Can you work these out from the model? Positions are in its coordinate system, mm. A direction names the side the tool comes from. Round coordinates to 2 decimals unless told otherwise and drop trailing zeros. Loops run counter-clockwise (first coordinate to the right, second up) from the corner with the lowest first, then second, coordinate; pieces in that order, holes last.
(1) Thinking about a two-plate mould opening in X: for faces 1 (the face through (-13, 3, -69.85)), 2 (the face through (-95.25, 3, -63)), 3 (the face through (82.55, 3, 67)), which applies, released by +X, released by -X, zero draft, split by the parting line, or undercut?
(2) If I drill on line 1 along Z through (x, y) = (-29.5, 5.5); line 2 along X through (y, z) = (4.25, -48.5), over which ranges is the centre line in solid material (lowest first)?
(3) I want a section at A-A on x = 79. Write out the boundary of the cut face in (y, z).
(4) I want a section at B-B on z = 24. Write out the boundary of the cut face in (x, y).
(5) Which directions (+Z, -Z, +X, -X, +Y, -Y) give clear straight access to the entire face, cutting with the end or side of a thin tool? Please do faces 4 (the face through (-69.85, 3, 67)), 5 (the face through (6.35, 3, -67)), 6 (the face through (92, 3, -19.05)), 7 (the face through (-92, 3, 31.75)).
(6) Will this pin go through, and if not, where does the flat tip stop? pin 1 Ø3 at (x, y) = (-29, 5.5) entering from +Z.
from build123d import *

# Parameters (mm, degrees)
SKETCH1_W                   = 190.5
SKETCH1_H                   = 139.7
BOSS_EXTRUDE1_DEPTH         = 6.35
SKETCH2_W                   = 12.7
SKETCH2_H                   = 12.7
CUT_EXTRUDE1_DEPTH          = 6.35
LPATTERN1_COUNT             = 4
LPATTERN1_PITCH             = 25.4
LPATTERN2_COUNT             = 4
LPATTERN2_PITCH             = 25.4
CIRPATTERN1_COUNT           = 2
CIRPATTERN1_COPY_1_SKETCH_W = 12.7
CIRPATTERN1_COPY_1_SKETCH_H = 12.7
CIRPATTERN1_COPY_1_DEPTH    = 6.35
CIRPATTERN1_COPY_2_SKETCH_W = 12.7
CIRPATTERN1_COPY_2_SKETCH_H = 12.7
CIRPATTERN1_COPY_2_DEPTH    = 6.35
CIRPATTERN1_COPY_3_SKETCH_W = 12.7
CIRPATTERN1_COPY_3_SKETCH_H = 12.7
CIRPATTERN1_COPY_3_DEPTH    = 6.35
CIRPATTERN1_COPY_4_SKETCH_W = 12.7
CIRPATTERN1_COPY_4_SKETCH_H = 12.7
CIRPATTERN1_COPY_4_DEPTH    = 6.35
CIRPATTERN1_COPY_5_SKETCH_W = 12.7
CIRPATTERN1_COPY_5_SKETCH_H = 12.7
CIRPATTERN1_COPY_5_DEPTH    = 6.35
CIRPATTERN1_COPY_6_SKETCH_W = 12.7
CIRPATTERN1_COPY_6_SKETCH_H = 12.7
CIRPATTERN1_COPY_6_DEPTH    = 6.35
SKETCH3_W                   = 12.7
SKETCH3_H                   = 12.7
CUT_EXTRUDE2_DEPTH          = 6.35
LPATTERN3_COUNT             = 3
LPATTERN3_PITCH             = 25.4
LPATTERN4_COUNT             = 3
LPATTERN4_PITCH             = 25.4
CIRPATTERN2_COUNT           = 2
CIRPATTERN2_COPY_1_SKETCH_W = 12.7
CIRPATTERN2_COPY_1_SKETCH_H = 12.7
CIRPATTERN2_COPY_1_DEPTH    = 6.35
CIRPATTERN2_COPY_2_SKETCH_W = 12.7
CIRPATTERN2_COPY_2_SKETCH_H = 12.7
CIRPATTERN2_COPY_2_DEPTH    = 6.35
CIRPATTERN2_COPY_3_SKETCH_W = 12.7
CIRPATTERN2_COPY_3_SKETCH_H = 12.7
CIRPATTERN2_COPY_3_DEPTH    = 6.35
CIRPATTERN2_COPY_4_SKETCH_W = 12.7
CIRPATTERN2_COPY_4_SKETCH_H = 12.7
CIRPATTERN2_COPY_4_DEPTH    = 6.35


with BuildPart() as part:
    # Sketch1 → Boss-Extrude1 (new body)
    with BuildSketch(Plane(origin=(0, 0, 0), x_dir=(1, 0, 0), z_dir=(0, 1, 0))):
        Rectangle(SKETCH1_W, SKETCH1_H)
    extrude(amount=BOSS_EXTRUDE1_DEPTH)

    # Sketch2 → Cut-Extrude1 (cut)
    with BuildSketch(Plane(origin=(0, 6.35, 0), x_dir=(1, 0, 0), z_dir=(0, 1, 0))):
        with Locations((0, 69.85)):
            Rectangle(SKETCH2_W, SKETCH2_H)
    cut_extrude1 = extrude(amount=-CUT_EXTRUDE1_DEPTH, mode=Mode.SUBTRACT)

    # LPattern1: Cut-Extrude1 ×4
    with Locations(*[(-i * LPATTERN1_PITCH, 0, 0) for i in range(1, LPATTERN1_COUNT)]):
        add(cut_extrude1, mode=Mode.SUBTRACT)

    # LPattern2: Cut-Extrude1 ×4
    with Locations(*[(i * LPATTERN2_PITCH, 0, 0) for i in range(1, LPATTERN2_COUNT)]):
        add(cut_extrude1, mode=Mode.SUBTRACT)

    # CirPattern1: Cut-Extrude1 ×2 about axis
    cirpattern1_axis = Axis((0, 0, 0), (0, 1, 0))
    for i in range(1, CIRPATTERN1_COUNT):
        add(cut_extrude1.rotate(cirpattern1_axis, i * 360 / CIRPATTERN1_COUNT), mode=Mode.SUBTRACT)

    # CirPattern1 copy 1 sketch → CirPattern1 copy 1 (cut)
    with BuildSketch(Plane(origin=(25.4, 6.35, 0), x_dir=(-1, 0, 0), z_dir=(0, 1, 0))):
        with Locations((0, 69.85)):
            Rectangle(CIRPATTERN1_COPY_1_SKETCH_W, CIRPATTERN1_COPY_1_SKETCH_H)
    extrude(amount=-CIRPATTERN1_COPY_1_DEPTH, mode=Mode.SUBTRACT)

    # CirPattern1 copy 2 sketch → CirPattern1 copy 2 (cut)
    with BuildSketch(Plane(origin=(50.8, 6.35, 0), x_dir=(-1, 0, 0), z_dir=(0, 1, 0))):
        with Locations((0, 69.85)):
            Rectangle(CIRPATTERN1_COPY_2_SKETCH_W, CIRPATTERN1_COPY_2_SKETCH_H)
    extrude(amount=-CIRPATTERN1_COPY_2_DEPTH, mode=Mode.SUBTRACT)

    # CirPattern1 copy 3 sketch → CirPattern1 copy 3 (cut)
    with BuildSketch(Plane(origin=(76.2, 6.35, 0), x_dir=(-1, 0, 0), z_dir=(0, 1, 0))):
        with Locations((0, 69.85)):
            Rectangle(CIRPATTERN1_COPY_3_SKETCH_W, CIRPATTERN1_COPY_3_SKETCH_H)
    extrude(amount=-CIRPATTERN1_COPY_3_DEPTH, mode=Mode.SUBTRACT)

    # CirPattern1 copy 4 sketch → CirPattern1 copy 4 (cut)
    with BuildSketch(Plane(origin=(-25.4, 6.35, 0), x_dir=(-1, 0, 0), z_dir=(0, 1, 0))):
        with Locations((0, 69.85)):
            Rectangle(CIRPATTERN1_COPY_4_SKETCH_W, CIRPATTERN1_COPY_4_SKETCH_H)
    extrude(amount=-CIRPATTERN1_COPY_4_DEPTH, mode=Mode.SUBTRACT)

    # CirPattern1 copy 5 sketch → CirPattern1 copy 5 (cut)
    with BuildSketch(Plane(origin=(-50.8, 6.35, 0), x_dir=(-1, 0, 0), z_dir=(0, 1, 0))):
        with Locations((0, 69.85)):
            Rectangle(CIRPATTERN1_COPY_5_SKETCH_W, CIRPATTERN1_COPY_5_SKETCH_H)
    extrude(amount=-CIRPATTERN1_COPY_5_DEPTH, mode=Mode.SUBTRACT)

    # CirPattern1 copy 6 sketch → CirPattern1 copy 6 (cut)
    with BuildSketch(Plane(origin=(-76.2, 6.35, 0), x_dir=(-1, 0, 0), z_dir=(0, 1, 0))):
        with Locations((0, 69.85)):
            Rectangle(CIRPATTERN1_COPY_6_SKETCH_W, CIRPATTERN1_COPY_6_SKETCH_H)
    extrude(amount=-CIRPATTERN1_COPY_6_DEPTH, mode=Mode.SUBTRACT)

    # Sketch3 → Cut-Extrude2 (cut)
    with BuildSketch(Plane(origin=(0, 6.35, 0), x_dir=(1, 0, 0), z_dir=(0, 1, 0))):
        with Locations((-95.25, 0)):
            Rectangle(SKETCH3_W, SKETCH3_H)
    cut_extrude2 = extrude(amount=-CUT_EXTRUDE2_DEPTH, mode=Mode.SUBTRACT)

    # LPattern3: Cut-Extrude2 ×3
    with Locations(*[(0, 0, -i * LPATTERN3_PITCH) for i in range(1, LPATTERN3_COUNT)]):
        add(cut_extrude2, mode=Mode.SUBTRACT)

    # LPattern4: Cut-Extrude2 ×3
    with Locations(*[(0, 0, i * LPATTERN4_PITCH) for i in range(1, LPATTERN4_COUNT)]):
        add(cut_extrude2, mode=Mode.SUBTRACT)

    # CirPattern2: Cut-Extrude2 ×2 about axis
    cirpattern2_axis = Axis((0, 0, 0), (0, 1, 0))
    for i in range(1, CIRPATTERN2_COUNT):
        add(cut_extrude2.rotate(cirpattern2_axis, i * 360 / CIRPATTERN2_COUNT), mode=Mode.SUBTRACT)

    # CirPattern2 copy 1 sketch → CirPattern2 copy 1 (cut)
    with BuildSketch(Plane(origin=(0, 6.35, 25.4), x_dir=(-1, 0, 0), z_dir=(0, 1, 0))):
        with Locations((-95.25, 0)):
            Rectangle(CIRPATTERN2_COPY_1_SKETCH_W, CIRPATTERN2_COPY_1_SKETCH_H)
    extrude(amount=-CIRPATTERN2_COPY_1_DEPTH, mode=Mode.SUBTRACT)

    # CirPattern2 copy 2 sketch → CirPattern2 copy 2 (cut)
    with BuildSketch(Plane(origin=(0, 6.35, 50.8), x_dir=(-1, 0, 0), z_dir=(0, 1, 0))):
        with Locations((-95.25, 0)):
            Rectangle(CIRPATTERN2_COPY_2_SKETCH_W, CIRPATTERN2_COPY_2_SKETCH_H)
    extrude(amount=-CIRPATTERN2_COPY_2_DEPTH, mode=Mode.SUBTRACT)

    # CirPattern2 copy 3 sketch → CirPattern2 copy 3 (cut)
    with BuildSketch(Plane(origin=(0, 6.35, -25.4), x_dir=(-1, 0, 0), z_dir=(0, 1, 0))):
        with Locations((-95.25, 0)):
            Rectangle(CIRPATTERN2_COPY_3_SKETCH_W, CIRPATTERN2_COPY_3_SKETCH_H)
    extrude(amount=-CIRPATTERN2_COPY_3_DEPTH, mode=Mode.SUBTRACT)

    # CirPattern2 copy 4 sketch → CirPattern2 copy 4 (cut)
    with BuildSketch(Plane(origin=(0, 6.35, -50.8), x_dir=(-1, 0, 0), z_dir=(0, 1, 0))):
        with Locations((-95.25, 0)):
            Rectangle(CIRPATTERN2_COPY_4_SKETCH_W, CIRPATTERN2_COPY_4_SKETCH_H)
    extrude(amount=-CIRPATTERN2_COPY_4_DEPTH, mode=Mode.SUBTRACT)


solid = part.part
Filled sheet:
1. face 1: zero draft
1. face 2: released by -X
1. face 3: undercut
2. line 1: z = -63.5 to 63.5
2. line 2: x = -88.9 to 88.9
3. outline: (0, -63.5) - (6.35, -63.5) - (6.35, 63.5) - (0, 63.5) - close
4. outline: (-88.9, 0) - (88.9, 0) - (88.9, 6.35) - (-88.9, 6.35) - close
5. face 4: +Z, +Y, -Y
5. face 5: -Z, +Y, -Y
5. face 6: +X, +Y, -Y
5. face 7: -X, +Y, -Y
6. pin 1: stops at z = 63.5
